Geometry: final body of the model. Coordinates: model frame, mm. A direction names the side the tool comes from. Round coordinates to 2 decimals unless told otherwise and drop trailing zeros. Write each loop counter-clockwise with the first axis right and the second up, starting at its lowest first coordinate (ties: lowest second). Pieces come first, ordered by that corner, then holes.
from build123d import *

# Parameters (mm, degrees)
PAD_DEPTH = 7
FILLET_R  = 3


with BuildPart() as part:
    # Sketch → Pad (new body)
    with BuildSketch(Plane.XY):
        Polygon((0, 0), (-40, 0), (-40, 3), (-25, 3), (-3, 25), (-3, 40), (0, 40), align=None)
        Polygon((-3, 22), (-22, 3), (-3, 3), align=None, mode=Mode.SUBTRACT)
    extrude(amount=PAD_DEPTH)

    # Fillet
    fillet_edges = [part.edges().sort_by_distance(p)[0] for p in [
        (-22, 3, 3.5),
        (-25, 3, 3.5),
        (-3, 22, 3.5),
        (-3, 25, 3.5),
        (-3, 3, 3.5),
    ]]
    fillet(fillet_edges, radius=FILLET_R)


solid = part.part
1) Section A-A on x = -12. Output: boundary loops of the cut face in (y, z).
2) Reachability of faces 1 (the flat face through (-3, 33, 3)), 2 (the flat face through (-20, 0, 3)), 3 (the cylindrical face through (-3.86, 3.9, 3.55)) from +Z, -Z, +X, -X, +Y, -Y: full face, straight path, thin tool, end or side. Return the list, or none.
3) Line query: probe 1 along X at (y, z) = (38.5, 2.75); probe 2 along X at (y, z) = (7, 1.75); probe 3 along Y at (x, z) = (-16, 0.5). Output: solid intervals per line, ascending.
4) Section D-D on x = -18.5. Output: boundary loops of the cut face in (y, z).
5) First-contact query: P1, Ø2, axis at x = -8, y = 5, coming from the +Z side; P2, Ø3, axis at x = -21.5, z = 3, coming from the -Y side; P3, Ø3.5, axis at x = -31, z = 5, coming from the +Y side; P4, Ø3.5, axis at y = 12.5, z = 4.5, coming from the -X side. Flat tips, straight axial feed; report the tip coordinate or a pass-through.
6) Section B-B on z = 4.25. Output: boundary loops of the cut face in (x, y).
7) Section C-C on y = 9.5. Output: boundary loops of the cut face in (x, z).
8) Draft query along Y for faces 4 (the flat face through (-14, 14, 3)), 5 (the flat face through (-40, 1, 3)), 6 (the flat face through (-3, 10, 3)). Return one class per face: pulls with the +Y half, pulls with the -Y half, needs draft (parallel to the pull), parting line crosses it, or undercut.
Filled in:
1. outline: (0, 0) - (3, 0) - (3, 7) - (0, 7) - close; (13, 0) - (16, 0) - (16, 7) - (13, 7) - close
2. face 1: +Z, -Z, -X, +Y
2. face 2: +Z, -Z, +X, -X, -Y
2. face 3: +Z, -Z
3. probe 1: x = -3 to 0
3. probe 2: x = -21 to -17.59, -3 to 0
3. probe 3: y = 0 to 3.27, 9 to 12
4. outline: (0, 0) - (9.5, 0) - (9.5, 7) - (0, 7) - close
5. P1: passes through
5. P2: stops at y = 0
5. P3: stops at y = 3
5. P4: stops at x = -17.25
6. outline: (-40, 0) - (0, 0) - (0, 40) - (-3, 40) - (-3, 26.24) arc R3 cw to (-3.88, 24.12) - (-24.12, 3.88) arc R3 cw to (-26.24, 3) - (-40, 3) - close; hole (-16.88, 8.12) arc R3 ccw to (-14.76, 3) - (-6, 3) arc R3 ccw to (-3, 6) - (-3, 14.76) arc R3 ccw to (-8.12, 16.88) - close
7. outline: (-18.5, 0) - (-15.5, 0) - (-15.5, 7) - (-18.5, 7) - close; (-3, 0) - (0, 0) - (0, 7) - (-3, 7) - close
8. face 4: pulls with the +Y half
8. face 5: needs draft
8. face 6: undercut
